from build123d import *

# Parameters (mm, degrees)
SKETCH_1_R          = 32.5
EXTRUDE_1_DEPTH     = 1.6
SKETCH_2_W          = 24
SKETCH_2_H          = 5.5
SKETCH_2_W_2        = 5.5
SKETCH_2_H_2        = 24
CUT_EXTRUDE_1_DEPTH = 1.6
SKETCH_3_R          = 0.8
CUT_EXTRUDE_2_DEPTH = 1.6
FILLET_1_R          = 1


with BuildPart() as part:
    # 草图1 → 凸台-拉伸1 (new body)
    with BuildSketch(Plane.XY):
        Circle(SKETCH_1_R)
    extrude(amount=EXTRUDE_1_DEPTH)

    # 草图2 → 切除-拉伸1 (cut)
    with BuildSketch(Plane.XY):
        with Locations((0, -29.75)):
            Rectangle(SKETCH_2_W, SKETCH_2_H)
        with Locations((29.75, 0)):
            Rectangle(SKETCH_2_W_2, SKETCH_2_H_2)
        with Locations((-29.75, 0)):
            Rectangle(SKETCH_2_W_2, SKETCH_2_H_2)
        with Locations((0, 29.75)):
            Rectangle(SKETCH_2_W, SKETCH_2_H)
    extrude(amount=CUT_EXTRUDE_1_DEPTH, mode=Mode.SUBTRACT)

    # 草图3 → 切除-拉伸2 (cut)
    with BuildSketch(Plane.XY.offset(1.6)):
        with Locations((21.25, 21.25)):
            Circle(SKETCH_3_R)
        with Locations((21.25, -21.25)):
            Circle(SKETCH_3_R)
        with Locations((-21.25, -21.25)):
            Circle(SKETCH_3_R)
        with Locations((-21.25, 21.25)):
            Circle(SKETCH_3_R)
    extrude(amount=-CUT_EXTRUDE_2_DEPTH, mode=Mode.SUBTRACT)

    # 圆角1
    fillet_1_edges = [part.edges().sort_by_distance(p)[0] for p in [
        (27, -12, 0.8),
        (27, 12, 0.8),
        (30.203476621, -12, 0.8),
        (30.203476621, 12, 0.8),
        (-12, -27, 0.8),
        (12, -30.203476621, 0.8),
        (12, -27, 0.8),
        (-12, -30.203476621, 0.8),
        (-27, 12, 0.8),
        (-30.203476621, -12, 0.8),
        (-27, -12, 0.8),
        (-30.203476621, 12, 0.8),
        (12, 27, 0.8),
        (-12, 30.203476621, 0.8),
        (-12, 27, 0.8),
        (12, 30.203476621, 0.8),
    ]]
    fillet(fillet_1_edges, radius=FILLET_1_R)


solid = part.part
Model file for the job. Use its own axes, mm. A direction names the side the tool comes from. Coordinates: 2 decimals unless noted, no trailing zeros. Order: outer loops, then holes, each group sorted by start corner. A loop starts at its lowest first (then second) coordinate and runs counter-clockwise, first axis right, second up. Notation, with made-up numbers: (-23, 48) -> (2, 48) arc R18 ccw to (2, 63) -> close; hole circle Ø10 at (46.25, 71.25). An arc over 180 degrees is marked (long way). Return JSON: item names as keys, results as strings. Group by question number.
Item 1: Wall check: line 1 along Y through (x, z) = (-21.25, 1.25); line 2 along X through (y, z) = (-1.5, 1.1). Give the ranges that are in metal, low to high. Write a range as [from, to].
Item 2: Saw through at D-D on y = 19.5. Write the cut outline in (x, z).
Item 3: Saw through at A-A on x = 21.25. Write the cut outline in (y, z), then the cut area to 3 significant figures.
Item 4: Saw through at C-C on z = 1.3. State how many separate pieces and enclosed holes the cut face has, then the cut area to 3 significant figures.
Item 5: Tool access for faces 1 (the flat face through (0, -27, 1)), 2 (the flat face through (-27, 0, 1)), 3 (the cylindrical face through (23.1, 22.86, 0.79)), 4 (the flat face through (27, 0, 1)): list every direction of +Z, -Z, +X, -X, +Y, -Y with a clear straight run to the whole face (end or side of a thin tool).
Item 6: Flat gauge pins, fed straight in: P1, Ø0.8, axis at x = 28.5, z = 0.5, coming from the -Y side; P2, Ø0.8, axis at x = -28.5, z = 1, coming from the +Y side; P3, Ø0.5, axis at y = 1, z = 0.5, coming from the -X side. Where does each tip first touch, or does it go through?
Item 7: Pull direction X, two halves, no side cores. Call faces 5 (the cylindrical face through (22.86, -23.1, 0.79)), 6 (the cylindrical face through (21.62, -21.96, 0.81)), 7 (the flat face through (0, 27, 1)), 8 (the cylindrical face through (-29.54, -12.47, 0.79)): pulls with the +X half, pulls with the -X half, needs draft (parallel to the pull), parting line crosses it, or undercut.
Values found:
{
 "1": {"line 1": "y = [-24.59, -22.05], [-20.45, 20.45], [22.05, 24.59]", "line 2": "x = [-27, 27]"},
 "2": {"outline": "(-26, 0) -> (26, 0) -> (26, 1.6) -> (-26, 1.6) -> close"},
 "3": {"outline": "(-24.59, 0) -> (-22.05, 0) -> (-22.05, 1.6) -> (-24.59, 1.6) -> close; (-20.45, 0) -> (20.45, 0) -> (20.45, 1.6) -> (-20.45, 1.6) -> close; (22.05, 0) -> (24.59, 0) -> (24.59, 1.6) -> (22.05, 1.6) -> close", "area": "73.6 mm2"},
 "4": {"separate pieces": "1", "enclosed holes": "4", "area": "2,850 mm2"},
 "5": {"face 1": "+Z, -Z, -Y", "face 2": "+Z, -Z, -X", "face 3": "+Z, -Z, +X, +Y", "face 4": "+Z, -Z, +X"},
 "6": {"P1": "stops at y = -16.33", "P2": "stops at y = 16.33", "P3": "stops at x = -27"},
 "7": {"face 5": "pulls with the +X half", "face 6": "undercut", "face 7": "undercut", "face 8": "pulls with the -X half"}
}
